Design review of the part built by this model. Coordinates are the model's own, in mm. A direction names the side the tool comes from. Round coordinates to 2 decimals unless told otherwise and drop trailing zeros. Write each loop counter-clockwise with the first axis right and the second up, starting at its lowest first coordinate (ties: lowest second). Pieces come first, ordered by that corner, then holes. Notation, with made-up numbers: (61.5, -20.5) - (120.5, -20.5) arc R22 cw to (120.5, 8.5) - close; hole circle Ø1 at (68, -29). An arc over 180 degrees is marked (long way). Use one line per item in the form item = value.
Autodesk Inventor part; units mm, degrees
ref_plane "Start Plane" through (0, 0, 0) normal (0, 0, 1) x (1, 0, 0)
ref_plane "End Plane" through (0, 0, 525) normal (0, 0, 1) x (1, 0, 0)
ref_plane "Work Plane4" through (21, 2290, 525) normal (0, 0, 1) x (1, 0, 0)
ref_plane "Start Plane" through (0, 0, 0) normal (0, 0, 1) x (1, 0, 0)
ref_plane "End Plane" through (0, 0, 525) normal (0, 0, 1) x (1, 0, 0)
sketch "Sketch" plane through (0, 0, 0) normal (0, 0, 1) x (1, 0, 0)
  line L0 (-25, -41) -> (-25, 41)
  line L1 (-21, 45) -> (21, 45)
  line L2 (25, 41) -> (25, -41)
  line L3 (21, -45) -> (-21, -45)
  arc A0 (-25, -41) -> (-21, -45) centre (-21, -41) ccw
  arc A1 (25, 41) -> (21, 45) centre (21, 41) ccw
  arc A2 (-21, 45) -> (-25, 41) centre (-21, 41) ccw
  arc A3 (21, -45) -> (25, -41) centre (21, -41) ccw
  arc A4 (-21, 43) -> (-23, 41) centre (-21, 41) ccw
  line L4 (-21, 43) -> (21, 43)
  arc A5 (23, 41) -> (21, 43) centre (21, 41) ccw
  line L5 (23, 41) -> (23, -41)
  arc A6 (21, -43) -> (23, -41) centre (21, -41) ccw
  line L6 (21, -43) -> (-21, -43)
  arc A7 (-23, -41) -> (-21, -43) centre (-21, -41) ccw
  line L7 (-23, -41) -> (-23, 41)
  line L8 (0, 64.1598) -> (0, -64.1598) construction
  line L9 (-36.1598, 0) -> (36.1598, 0) construction
  dimension "d7" = 4
  dimension "d9" = 50
  dimension "d11" = 90
  dimension "d12" = 2
  dimension "d15" = 25
  dimension "d16" = 45
extrude "Body" add sketch "Sketch" along normal up to surface (525 mm away) from surface at 0
sketch "Sketch3" plane through (0, 0, 0) normal (0, 0, 1) x (1, 0, 0)
  line L0 (0, 0) -> (10, 0)
ref_plane "Work Plane3" through (0, 0, 0) normal (0, -1, 0) x (1, 0, 0)
sketch "Sketch4" plane through (0, 0, 0) normal (0, -1, 0) x (1, 0, 0)
  line L0 (-2, 0) -> (12, 0)
  line L1 (-2, 525) -> (12, 525)
  dimension "d18" = 525
ref_plane "Work Plane4" through (21, 2290, 525) normal (0, 0, 1) x (1, 0, 0)
split "Split1" plane through (21, 2290, 525) removes the side toward (0, 0, 1)
sketch "Sketch5" plane through (-25, 41, 0) normal (-1, 0, 0) x (0, 0, 1)
  line L0 (395, -21) -> (455, -21)
  line L1 (455, -21) -> (455, -61)
  line L2 (455, -61) -> (395, -61)
  line L3 (395, -61) -> (395, -21)
  line L4 (525, -82) -> (525, 0)
  line L5 (525, -41) -> (516.5048, -41)
  point P0 (0, -41)
  dimension "d19" = 60
  dimension "d20" = 40
  dimension "d21" = 70
hole "Hole1" at (-25, 20, 395) at (-25, -20, 395) at (-25, 20, 455) at (-25, -20, 455) direction (1, 0, 0) diameter 6.8 end through all
equation "\"d7\" = G_IR"
equation "\"d9\" = G_W"
equation "\"d11\" = G_H"
equation "\"d12\" = G_T"
equation "\"d15\" = 0.5 * d9"
equation "\"d16\" = 0.5 * d11"
equation "\"d3\" = G_L"
equation "\"G_W\" = 50"
equation "\"G_H\" = 90"
equation "\"G_T\" = 2"
equation "\"G_IR\" = 4"
equation "\"G_L\" = d18"
equation "\"G_OFFSET_START\" = 0"
equation "\"G_OFFSET_END\" = -25"
equation "\"d14\" = G_OFFSET_END + B_L"
properties part number "ISO 10799-2 - 90x50x2 - 525" material "Steel, Mild"
Q1. To check wall thickness, follow line 1 along Z through (x, y) = (24.5, 20); line 2 along X through (y, z) = (32, 300.5); line 3 along Y through (x, z) = (3.5, 402.5). State the ranges of each line that lie inside material, in increasing order. Write a range as from..to.
Calculated:
line_1 = 0..391.6, 398.4..451.6, 458.4..525
line_2 = -25..-23, 23..25
line_3 = -45..-43, 43..45
Q2. We need section A-A on x = 3. Write out the cut boundary in (y, z), then the cut area to 3 significant figures.
Calculated:
outline = (-45, 0) - (-43, 0) - (-43, 525) - (-45, 525) - close; (43, 0) - (45, 0) - (45, 525) - (43, 525) - close
area = 2,100 mm2
Q3. We need section B-B on z = 39. Write out the cut boundary in (x, y), then the cut area to 3 significant figures.
Calculated:
outline = (-25, -41) arc R4 ccw to (-21, -45) - (21, -45) arc R4 ccw to (25, -41) - (25, 41) arc R4 ccw to (21, 45) - (-21, 45) arc R4 ccw to (-25, 41) - close; hole (-23, -41) arc R2 ccw to (-21, -43) - (21, -43) arc R2 ccw to (23, -41) - (23, 41) arc R2 ccw to (21, 43) - (-21, 43) arc R2 ccw to (-23, 41) - close
area = 534 mm2
Q4. Draft analysis for pull direction Y (two halves, no side actions). For faces 3 (the flat face through (0, 43, 259)), 4 (the flat face through (0, 45, 259)), 5 (the flat face through (25, 1, 259)), 6 (the flat face through (23, 1, 259)), state which applies: released by +Y, released by -Y, zero draft, split by the parting line, or undercut.
Calculated:
face_3 = undercut
face_4 = released by +Y
face_5 = zero draft
face_6 = undercut
Q5. Machinability: for faces 1 (the flat face through (0, -45, 259)), 2 (the flat face through (0, -43, 259)), which of the approach directions +Z, -Z, +X, -X, +Y, -Y give a long, thin tool a straight path to every point of the face, cutting with its end or side? Answer none if there is none.
Calculated:
face_1 = +Z, -Z, +X, -X, -Y
face_2 = +Z, -Z
